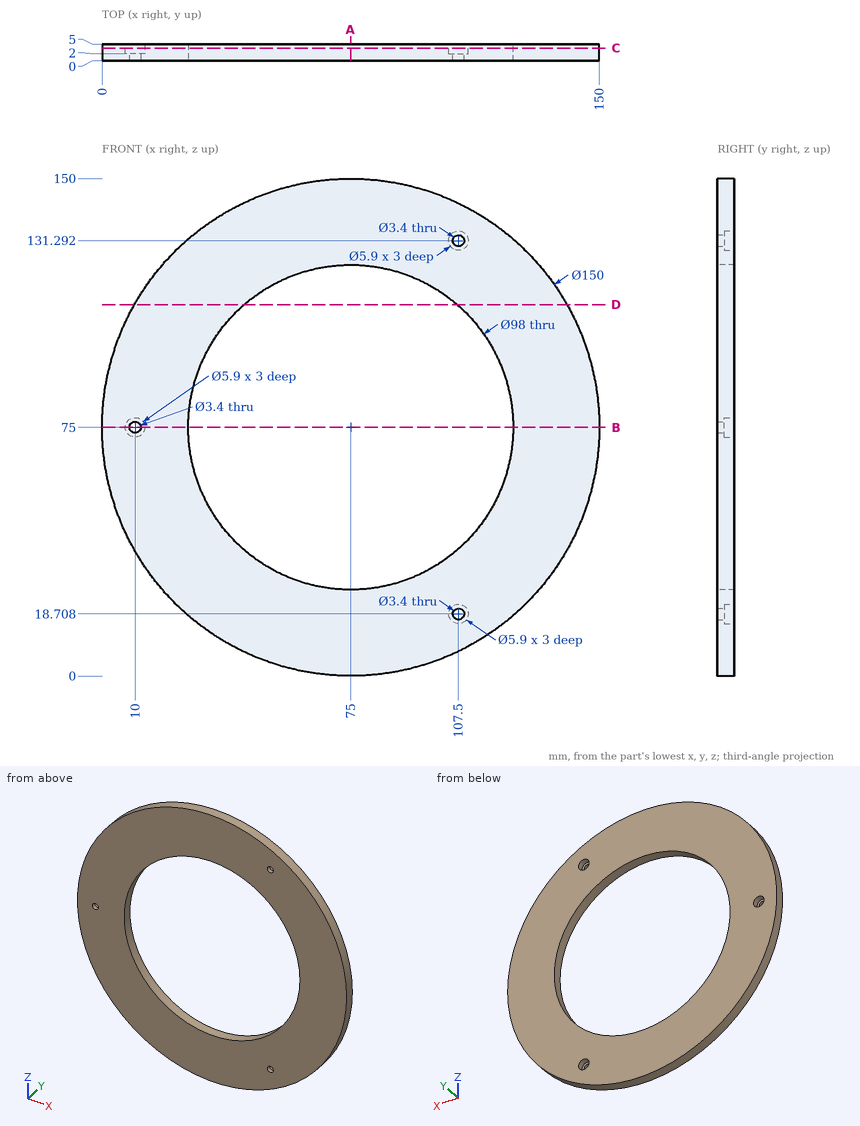
Here's the drawing with two shaded views (mm, measured from the low corner). I have some questions. Coordinates: 2 decimals unless noted, no trailing zeros. Order: outer loops, then holes, each group sorted by start corner. A loop starts at its lowest first (then second) coordinate and runs counter-clockwise, first axis right, second up. Notation, with made-up numbers: (81.5, 56.5) - (96.5, 56.5) arc R19 cw to (96.5, 70.5) - close; hole circle Ø6 at (84.5, 32). An arc over 180 degrees is marked (long way). Answer in a Markdown table with one row per item.
1. If I drill on line 1 along X through (y, z) = (3.25, 75); line 2 along Z through (x, y) = (107.5, 1.5); line 3 along Z through (x, y) = (75, 2.35), over which ranges is the centre line in solid material (lowest first)?
Reply:
| item | result |
|---|---|
| line 1 | x = 0 to 7.05, 12.95 to 26, 124 to 150 |
| line 2 | z = 7.41 to 17.01, 20.41 to 38.33, 111.67 to 129.59, 132.99 to 142.59 |
| line 3 | z = 0 to 26, 124 to 150 |
2. For pin 1 (3 mm diameter, centred on x = 19.5, y = 3.5, fed in from -Z); pin 2 (1 mm diameter, centred on y = 2, z = 15, fed in from -X), each with a flat end and sliding along its axis, tell me the tip position at first contact or that it passes through.
Reply:
| item | result |
|---|---|
| pin 1 | stops at z = 22.95 |
| pin 2 | stops at x = 29.34 |
3. Suppose I cut it at D-D (z = 112). Please give me the cut outline in (x, y) (1 decimal).
Reply:
| item | result |
|---|---|
| outline | (9.8, 0) - (42.9, 0) - (42.9, 5) - (9.8, 5) - close; (107.1, 0) - (140.2, 0) - (140.2, 5) - (107.1, 5) - close |
4. Suppose I cut it at A-A (x = 75). Please give me the cut outline in (y, z).
Reply:
| item | result |
|---|---|
| outline | (0, 0) - (5, 0) - (5, 26) - (0, 26) - close; (0, 124) - (5, 124) - (5, 150) - (0, 150) - close |
5. Suppose I cut it at C-C (y = 3.75). Give the number of separate pieces and of enclosed holes in the cut face, and give its area (3 significant figures).
Reply:
| item | result |
|---|---|
| separate pieces | 1 |
| enclosed holes | 4 |
| area | 10,000 mm^2 |
6. Suppose I cut it at B-B (z = 75). Please give me the cut outline in (x, y).
Reply:
| item | result |
|---|---|
| outline | (0, 0) - (8.3, 0) - (8.3, 2) - (7.05, 2) - (7.05, 5) - (0, 5) - close; (11.7, 0) - (26, 0) - (26, 5) - (12.95, 5) - (12.95, 2) - (11.7, 2) - close; (124, 0) - (150, 0) - (150, 5) - (124, 5) - close |
